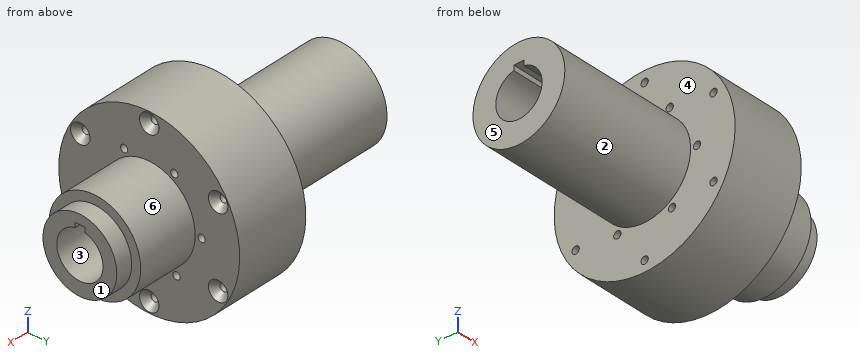
from build123d import *

# Parameters (mm, degrees)
F2_DEPTH       = 25
F4_D           = 5
F4_CSINK_D     = 13.44
F4_CSINK_ANGLE = 90
F6_D           = 5
F8_DEPTH       = 201.5


with BuildPart() as f1:
    # F0 (on Front) → F1 (revolve)
    with BuildSketch(Plane.XZ):
        Polygon((-272.2911421515, 31.75), (-272.2911421515, 16), (-70.7911421515, 16), (-70.7911421515, 25.5), (-82.2911421515, 25.5), (-82.2911421515, 31.75), (-149.2911421515, 31.75), (-149.2911421515, 62.5), (-175.2911421515, 62.5), (-175.2911421515, 31.75), align=None)
    revolve(axis=Axis((18.6580618019, 0, 0), (1, 0, 0)))

    # F2 (add): a face of the model
    f2_faces = [f1.faces().sort_by_distance(p)[0] for p in [
        (-149.2911421515, 0, -33.517766953),
    ]]
    extrude(f2_faces, amount=F2_DEPTH)

    # F4 (through all)
    with Locations(Plane.YZ.offset(-124.2911421515)):
        with Locations((-47.6313972081, 27.5), (47.6313972081, 27.5), (0, 55), (0, -55), (47.6313972081, -27.5), (-47.6313972081, -27.5)):
            CounterSinkHole(F4_D / 2, F4_CSINK_D / 2, counter_sink_angle=F4_CSINK_ANGLE)

    # F6 (through all)
    with Locations(Plane.YZ.offset(-124.2911421515)):
        with Locations((-36.2002509452, 0), (-17.3218229571, 31.7869881861), (17.3218229571, 31.7869881861), (36.2002509452, 0), (18.8674278004, -30.8946328137), (-18.8674278004, -30.8946328137)):
            Hole(F6_D / 2)

    # F7 (on face) → F8 (cut, through all)
    with BuildSketch(Plane.YZ.offset(-70.7911421515)):
        with BuildLine():
            ThreePointArc((-3.5, 15.612494996), (0, 16), (3.5, 15.612494996))
            Line((3.5, 15.612494996), (3.5, 19))
            Line((3.5, 19), (-3.5, 19))
            Line((-3.5, 19), (-3.5, 15.612494996))
        make_face()
    extrude(amount=-F8_DEPTH, mode=Mode.SUBTRACT)


solid = f1.part
Geometry: final body of the model. Coordinates: model frame, mm. Face numbers are marked on the shaded views. A direction names the side the tool comes from. Round coordinates to 2 decimals unless told otherwise and drop trailing zeros. Loops run counter-clockwise (first coordinate to the right, second up) from the corner with the lowest first, then second, coordinate; pieces in that order, holes last.
Q1. Material intervals for L1, parallel to Y at x = -146, z = 27; L2, parallel to Y at x = -156, z = 27.5; L3, parallel to X at y = -30, z = -20, sorted ascending.
Q2. Section C-C on z = -55. Return loops of the section in (x, y).
Q3. Pin query (flat end, axial travel): P1, Ø3, axis at y = -47.63, z = -27.5, coming from the -X side; P2, Ø5, axis at y = -16, z = -35.5, coming from the -X side; P3, Ø6.5, axis at y = 0, z = -55, coming from the +X side; P4, Ø6, axis at y = 18.87, z = -30.89, coming from the +X side. Return the tip coordinate at first contact, or that it passes through.
Q4. Section B-B on y = 0. State how many separate pieces and enclosed holes the cut face has, plus the area to 3 significant figures.
Q5. Section A-A on z = 0. Return loops of the section in (x, y).
Q6. Pull-direction query (Y, two-part tool) for the marked faces 1, 2 and 3; classes: released by +Y, released by -Y, zero draft, split by the parting line, or undercut.
Q7. Access query for the marked faces 4, 5 and 6. Directions: +Z, -Z, +X, -X, +Y, -Y. A direction counts if a zero-diameter tool reaches every point of the face in a straight line with its end or side. Return the directions, or none.
Evaluation:
1. L1: y = -56.37 to -50.08, -45.18 to 45.18, 50.08 to 56.37
1. L2: y = -56.12 to -50.13, -45.13 to 45.13, 50.13 to 56.12
1. L3: x = -175.29 to -124.29
2. outline: (-175.29, -29.69) - (-124.29, -29.69) - (-124.29, -6.72) - (-128.51, -2.5) - (-175.29, -2.5) - close; (-175.29, 2.5) - (-128.51, 2.5) - (-124.29, 6.72) - (-124.29, 29.69) - (-175.29, 29.69) - close
3. P1: passes through
3. P2: stops at x = -175.29
3. P3: stops at x = -127.76
3. P4: stops at x = -124.29
4. separate pieces: 4
4. enclosed holes: 0
4. area: 8,190 mm2
5. outline: (-272.29, -31.75) - (-175.29, -31.75) - (-175.29, -33.7) - (-124.29, -33.7) - (-124.29, -31.75) - (-82.29, -31.75) - (-82.29, -25.5) - (-70.79, -25.5) - (-70.79, -16) - (-272.29, -16) - close; (-272.29, 16) - (-70.79, 16) - (-70.79, 25.5) - (-82.29, 25.5) - (-82.29, 31.75) - (-124.29, 31.75) - (-124.29, 33.7) - (-175.29, 33.7) - (-175.29, 31.75) - (-272.29, 31.75) - close; (-175.29, -62.5) - (-124.29, -62.5) - (-124.29, -38.7) - (-175.29, -38.7) - close; (-175.29, 38.7) - (-124.29, 38.7) - (-124.29, 62.5) - (-175.29, 62.5) - close
6. face 1: zero draft
6. face 2: split by the parting line
6. face 3: undercut
7. face 4: -X
7. face 5: +Z, -Z, -X, +Y, -Y
7. face 6: +X
